```python
from build123d import *

# Parameters (mm, degrees)
SKETCH2_W = 19.8
SKETCH2_H = 2.5
FILLET1_R = 0.762
FILLET2_R = 0.254


with BuildPart() as part:
    # Sketch1 → Flange (revolve)
    with BuildSketch(Plane(origin=(0, 0, 0), x_dir=(0, 0, -1), z_dir=(1, 0, 0)), mode=Mode.PRIVATE) as flange_sk:
        Polygon((-37.5, 0), (-37.5, 3.175), (-30.315802195, 5.1), (0, 5.1), (0, 2.5), (-26.1, 2.5), (-26.1, 0), align=None)
    revolve(flange_sk.sketch.rotate(Axis((0, 0, 0), (0, 1, 0)), 180), axis=Axis((0, 0, 0), (0, 1, 0)))

    # Sketch2 → Blank Insert (revolve)
    with BuildSketch(Plane(origin=(0, 0, 0), x_dir=(0, 0, -1), z_dir=(1, 0, 0))):
        with Locations((-9.9, 1.25)):
            Rectangle(SKETCH2_W, SKETCH2_H)
    revolve(axis=Axis((0, 0, 0), (0, -1, 0)))

    # Fillet1
    fillet1_edges = [part.edges().sort_by_distance(p)[0] for p in [
        (0, 3.175, 37.5),
    ]]
    fillet(fillet1_edges, radius=FILLET1_R)

    # Fillet2
    fillet2_edges = [part.edges().sort_by_distance(p)[0] for p in [
        (0, 0, 37.5),
    ]]
    fillet(fillet2_edges, radius=FILLET2_R)


solid = part.part
```
Geometry check sheet. Reference: the model listing, model coordinates, mm. A direction names the side the tool comes from. Round coordinates to 2 decimals unless told otherwise and drop trailing zeros. Loops run counter-clockwise (first coordinate to the right, second up) from the corner with the lowest first, then second, coordinate; pieces in that order, holes last. Notation, with made-up numbers: M -4.75,58.5 L 31.25,58.5 A20 ccw 31.25,83.5 Z; hole C -14,60.5 d6. An arc over 180 degrees is marked long. Return JSON: item names as keys, results as strings. Group by question number.
(1) Go/stop test with flat-tipped pins: pin 1 (1 mm diameter, centred on x = 1, y = 3.5, fed in from -Z); pin 2 (2 mm diameter, centred on x = -3.5, y = 3.5, fed in from +Z). Record where each tip stops, or that it passes through.
(2) Section check A-A, the plane y = 1.3. Enter the section's corners in (x, z).
(3) Set-up check for faces 4 (the face through (-5.9, 1.3, 18.9)), 5 (the face through (0, 0, 0)): record each of +Z, -Z, +X, -X, +Y, -Y from which the full face is reachable in a straight line by a thin tool's end or side.
(4) Scan lines: line 1 along X through (y, z) = (1.3, 0); line 2 along Z through (x, y) = (9, 1.25); line 3 along Z through (x, y) = (-1.5, 1). Record each from-to range of solid material in increasing order. Write a range as [from, to].
(5) Mould release check, pull along X, two halves, no side actions. Record for faces 1 (the face through (-25.4, 0, 7.8)), 2 (the face through (-9.203, 5.014, -29.222)), 3 (the face through (-18, 2.5, 10)): pulls with the +X half, pulls with the -X half, needs draft (parallel to the pull), parting line crosses it, or undercut.
Data:
{
 "1": {"pin 1": "z = -37.37", "pin 2": "z = 37.38"},
 "2": {"outline": "C 0,0 d75; C 0,0 d39.6; hole C 0,0 d52.2"},
 "3": {"face 4": "-Y", "face 5": "+Z, -Z, +X, -X, -Y"},
 "4": {"line 1": "[-37.5, -26.1], [-19.8, 19.8], [26.1, 37.5]", "line 2": "[-36.4, -24.5], [-17.64, 17.64], [24.5, 36.4]", "line 3": "[-37.47, -26.06], [-19.74, 19.74], [26.06, 37.47]"},
 "5": {"face 1": "needs draft", "face 2": "parting line crosses it", "face 3": "undercut"}
}
